from build123d import *

# Parameters (mm, degrees)
BOSS_EXTRUDE1_DEPTH = 32
SKETCH3_W           = 20
SKETCH3_H           = 12.2
BOSS_EXTRUDE2_DEPTH = 4.5
SKETCH4_R           = 3.5
CUT_EXTRUDE1_DEPTH  = 34
SKETCH5_R           = 3.5
CUT_EXTRUDE2_DEPTH  = 9
FILLET1_R           = 2.5


with BuildPart() as part:
    # Sketch1 → Boss-Extrude1 (new body)
    with BuildSketch(Plane(origin=(0, 0, 0), x_dir=(1, 0, 0), z_dir=(0, 1, 0))):
        with BuildLine():
            Line((-16.5, 10), (16.5, 10))
            Line((16.5, 10), (16.5, -10))
            ThreePointArc((16.5, -10), (0, -12.313346431), (-16.5, -10))
            Line((-16.5, -10), (-16.5, 10))
        make_face()
    extrude(amount=BOSS_EXTRUDE1_DEPTH)

    # Sketch3 → Boss-Extrude2 (add)
    with BuildSketch(Plane.ZY.offset(16.5)):
        with Locations((0, -6.1)):
            Rectangle(SKETCH3_W, SKETCH3_H)
    boss_extrude2 = extrude(amount=-BOSS_EXTRUDE2_DEPTH)

    # Mirror1: Boss-Extrude2 across plane
    add(boss_extrude2.mirror(Plane(origin=(0, 0, 0), x_dir=(0, 0, 1), z_dir=(1, 0, 0))))

    # Sketch4 → Cut-Extrude1 (cut, through all)
    with BuildSketch(Plane.ZY.offset(16.5)):
        with Locations((0, -7.2)):
            Circle(SKETCH4_R)
    extrude(amount=-CUT_EXTRUDE1_DEPTH, mode=Mode.SUBTRACT)

    # Sketch5 → Cut-Extrude2 (cut)
    with BuildSketch(Plane.ZY.offset(16.5)):
        with Locations((0, 24.5)):
            Circle(SKETCH5_R)
    extrude(amount=-CUT_EXTRUDE2_DEPTH, mode=Mode.SUBTRACT)

    # Fillet1
    fillet1_edges = [part.edges().sort_by_distance(p)[0] for p in [
        (-12, -6.1, -10),
        (12, -6.1, -10),
    ]]
    fillet(fillet1_edges, radius=FILLET1_R)


solid = part.part
The listing builds one solid part. Answer for the finished solid, in the listing's coordinates (mm). A direction names the side the tool comes from. Round coordinates to 2 decimals unless told otherwise and drop trailing zeros. Write each loop counter-clockwise with the first axis right and the second up, starting at its lowest first coordinate (ties: lowest second). Pieces come first, ordered by that corner, then holes. Notation, with made-up numbers: (60, 71.5) - (96, 71.5) arc R25 ccw to (96, 89.5) - close; hole circle Ø8 at (21, -21.75). An arc over 180 degrees is marked (long way). Use one line per item in the form item = value. Start each with the question number.
Item 1: A cutting plane is placed at A-A (y = -2.5). Write down the section's boundary in (x, z).
Item 2: A tool of negligible diameter and unlimited length cuts with its end or side. For faces 1 (the flat face through (-7.5, 25, 0)), 2 (the cylindrical face through (-12.752, -6.015, -9.287)), 3 (the flat face through (14, -6, 10)), 4 (the flat face through (-12, -5, 3)), from which of +Z, -Z, +X, -X, +Y, -Y can it reach the whole face along a straight path? Write none if from no direction.
Item 3: A cutting plane is placed at D-D (z = 4). Write down the section's boundary in (x, y).
Item 4: Find the intervals of material crossed by line 1 (Y direction, x = -13.6, z = 0); line 2 (X direction, y = -5, z = 3.75); line 3 (Z direction, x = 15, y = -7), in increasing order. Write a range as [from, to].
Item 5: Flat-ended cylindrical pins translate along their axes: pin 1 Ø2 at (x, z) = (-5.5, 1) entering from -Y; pin 2 Ø5.5 at (y, z) = (-7.2, 0) entering from +X; pin 3 Ø2 at (x, y) = (14.5, -7.5) entering from +Z; pin 4 Ø10 at (y, z) = (-5.5, 0) entering from +X. Find the tip coordinate at first contact, or state that the pin passes through.
Item 6: Determine the mould class of faces 5 (the flat face through (14, -12.2, 0)), 6 (the cylindrical face through (12.752, -6.015, -9.287)), 7 (the cylindrical face through (14.22, -3.73, -0.46)) for opening direction Y: +Y half, -Y half, draft (parallel to the pull), parting line (faces both ways), or undercut.
Item 7: A cutting plane is placed at C-C (z = 1). Write down the section's boundary in (x, y).
Item 8: A cutting plane is placed at B-B (y = -7.2). Write down the section's boundary in (x, z).
The answers:
q1.outline = (-16.5, -10) - (-14.5, -10) arc R2.5 ccw to (-12, -7.5) - (-12, 10) - (-16.5, 10) - close; (12, -7.5) arc R2.5 ccw to (14.5, -10) - (16.5, -10) - (16.5, 10) - (12, 10) - close
q2.face_1 = -X
q2.face_2 = -Z, -Y
q2.face_3 = +Z, +X, -X, -Y
q2.face_4 = +Z, -Z, -Y
q3.outline = (-16.5, -12.2) - (-12, -12.2) - (-12, 0) - (12, 0) - (12, -12.2) - (16.5, -12.2) - (16.5, 32) - (-16.5, 32) - close
q4.line_1 = [-12.2, -10.7], [-3.7, 21], [28, 32]
q4.line_2 = [-16.5, -12], [12, 16.5]
q4.line_3 = [-10, -3.49], [3.49, 10]
q5.pin_1 = 0
q5.pin_2 = through
q5.pin_3 = 10
q5.pin_4 = 16.5
q6.face_5 = -Y half
q6.face_6 = draft
q6.face_7 = undercut
q7.outline = (-16.5, -12.2) - (-12, -12.2) - (-12, -10.55) - (-16.5, -10.55) - close; (-16.5, -3.85) - (-12, -3.85) - (-12, 0) - (12, 0) - (12, -3.85) - (16.5, -3.85) - (16.5, 32) - (-16.5, 32) - (-16.5, 27.85) - (-7.5, 27.85) - (-7.5, 21.15) - (-16.5, 21.15) - close; (12, -12.2) - (16.5, -12.2) - (16.5, -10.55) - (12, -10.55) - close
q8.outline = (-16.5, -10) - (-14.5, -10) arc R2.5 ccw to (-12, -7.5) - (-12, -3.5) - (-16.5, -3.5) - close; (-16.5, 3.5) - (-12, 3.5) - (-12, 10) - (-16.5, 10) - close; (12, -7.5) arc R2.5 ccw to (14.5, -10) - (16.5, -10) - (16.5, -3.5) - (12, -3.5) - close; (12, 3.5) - (16.5, 3.5) - (16.5, 10) - (12, 10) - close
